from build123d import *

# Parameters (mm, degrees)
F1_DEPTH = 1.27
F2_DEPTH = 8.89
F3_R     = 5.715
F3_R_2   = 2.9972
F4_DEPTH = 1.27
F5_R     = 6.35
F5_R_2   = 2.9972
F6_DEPTH = 1.27


with BuildPart() as f1:
    # F0 (on Front) → F1 (new body)
    with BuildSketch(Plane.XZ):
        with BuildLine():
            ThreePointArc((7.62, 0), (5.388154, 5.388154), (0, 7.62))
            Line((0, 7.62), (0, 6.35))
            Line((0, 6.35), (3.683, 6.35))
            Line((3.683, 6.35), (7.315638, 0))
            Line((7.315638, 0), (7.62, 0))
        make_face()
        with BuildLine():
            Line((0, 6.35), (0, 7.62))
            ThreePointArc((0, 7.62), (-5.388154, 5.388154), (-7.62, 0))
            Line((-7.62, 0), (-7.315638, 0))
            Line((-7.315638, 0), (-3.683, 6.35))
            Line((-3.683, 6.35), (0, 6.35))
        make_face()
        with BuildLine():
            ThreePointArc((0, -7.62), (5.388154, -5.388154), (7.62, 0))
            Line((7.62, 0), (7.315638, 0))
            Line((7.315638, 0), (3.683, -6.35))
            Line((3.683, -6.35), (0, -6.35))
            Line((0, -6.35), (0, -7.62))
        make_face()
        with BuildLine():
            Line((-7.315638, 0), (-7.62, 0))
            ThreePointArc((-7.62, 0), (-5.388154, -5.388154), (0, -7.62))
            Line((0, -7.62), (0, -6.35))
            Line((0, -6.35), (-3.683, -6.35))
            Line((-3.683, -6.35), (-7.315638, 0))
        make_face()
    extrude(amount=F1_DEPTH)

    # F0 (on Front) → F2 (join)
    with BuildSketch(Plane.XZ):
        with BuildLine():
            Line((3.683, 6.35), (0, 6.35))
            Line((0, 6.35), (0, 2.9972))
            ThreePointArc((0, 2.9972), (2.11934, 2.11934), (2.9972, 0))
            Line((2.9972, 0), (7.315638, 0))
            Line((7.315638, 0), (3.683, 6.35))
        make_face()
        with BuildLine():
            Line((0, 2.9972), (0, 6.35))
            Line((0, 6.35), (-3.683, 6.35))
            Line((-3.683, 6.35), (-7.315638, 0))
            Line((-7.315638, 0), (-2.9972, 0))
            ThreePointArc((-2.9972, 0), (-2.11934, 2.11934), (0, 2.9972))
        make_face()
        with BuildLine():
            Line((-2.9972, 0), (-7.315638, 0))
            Line((-7.315638, 0), (-3.683, -6.35))
            Line((-3.683, -6.35), (0, -6.35))
            Line((0, -6.35), (0, -2.9972))
            ThreePointArc((0, -2.9972), (-2.11934, -2.11934), (-2.9972, 0))
        make_face()
        with BuildLine():
            Line((3.683, -6.35), (7.315638, 0))
            Line((7.315638, 0), (2.9972, 0))
            ThreePointArc((2.9972, 0), (2.11934, -2.11934), (0, -2.9972))
            Line((0, -2.9972), (0, -6.35))
            Line((0, -6.35), (3.683, -6.35))
        make_face()
    extrude(amount=F2_DEPTH)

    # F3 (on face) → F4 (join)
    with BuildSketch(Plane.XZ.offset(8.89)):
        Circle(F3_R)
        Circle(F3_R_2, mode=Mode.SUBTRACT)
    extrude(amount=F4_DEPTH)

    # F5 (on face) → F6 (join)
    with BuildSketch(Plane.XZ.offset(10.16)):
        Circle(F5_R)
        Circle(F5_R_2, mode=Mode.SUBTRACT)
    extrude(amount=F6_DEPTH)


solid = f1.part
Geometry check sheet. Reference: the model listing, model coordinates, mm. A direction names the side the tool comes from. Give positions to 0.01 mm unless a question says otherwise; leave off trailing zeros. Write each loop counter-clockwise with the first axis right and the second up, starting at its lowest first coordinate (ties: lowest second). Pieces come first, ordered by that corner, then holes. Notation, with made-up numbers: M 61.25,-31 L 68.25,-31 A21 ccw 68.25,-22 Z; hole C 23.5,35.5 d10. An arc over 180 degrees is marked long. Answer as CSV lines item,"result". Start each with the question number.
Q1. Go/stop test with flat-tipped pins: pin 1 (2 mm diameter, centred on x = 6, y = -1.5, fed in from -Z); pin 2 (3.5 mm diameter, centred on x = 0, y = -4, fed in from +Z); pin 3 (4 mm diameter, centred on y = -4.5, z = 5.5, fed in from -X). Record where each tip stops, or that it passes through.
Q2. Section check D-D, the plane x = 4.5. Record the cut outline in (y, z).
Q3. Section check B-B, the plane z = -1. Record the cut outline in (x, y), then the cut area to 3 significant figures.
Q4. Section check C-C, the plane x = 2.5. Record the cut outline in (y, z), then the cut area to 3 significant figures.
Q5. Material ranges on L1, parallel to Y at x = -5.75, z = -1.5; L2, parallel to Z at x = 0, y = -9.5 (3 decimals); L3, parallel to Z at x = 0, y = -10.85, recorded low to high.
Q6. Release check for a two-part mould opening along Y. For faces 4 (the face through (3, -11.43, -1)), 5 (the face through (4.84, -8.89, 3.32)), 6 (the face through (5.45, -9.52, 1.72)), 7 (the face through (0, -5, -6.35)) record: pulls with the +Y half, pulls with the -Y half, needs draft (parallel to the pull), parting line crosses it, or undercut.
Q7. Tool access check on faces 1 (the face through (-5.474, -5.027, 3.219)), 2 (the face through (-1.38, -10.79, -6.2)), 3 (the face through (5.525, -5.027, 3.131)). Record the directions out of +Z, -Z, +X, -X, +Y, -Y that give a thin tool (end or side, any length) a straight path to the whole face; none if there is none.
Q8. Section check A-A, the plane y = -1. Record the cut outline in (x, z).
Geometry says:
1,pin 1,"z = -5.73"
1,pin 2,"z = 6.35"
1,pin 3,"x = -5.31"
2,outline,"M -11.43,-4.48 L -10.16,-4.48 L -10.16,-3.52 L -8.89,-3.52 L -8.89,-4.92 L -1.27,-4.92 L -1.27,-6.15 L 0,-6.15 L 0,6.15 L -1.27,6.15 L -1.27,4.92 L -8.89,4.92 L -8.89,3.52 L -10.16,3.52 L -10.16,4.48 L -11.43,4.48 Z"
3,outline,"M -7.55,-1.27 L -6.74,-1.27 L -6.74,-8.89 L -5.63,-8.89 L -5.63,-10.16 L -6.27,-10.16 L -6.27,-11.43 L -2.83,-11.43 L -2.83,0 L -7.55,0 Z; M 2.83,-11.43 L 6.27,-11.43 L 6.27,-10.16 L 5.63,-10.16 L 5.63,-8.89 L 6.74,-8.89 L 6.74,-1.27 L 7.55,-1.27 L 7.55,0 L 2.83,0 Z"
3,area,"87.6 mm^2"
4,outline,"M -11.43,-5.84 L -10.16,-5.84 L -10.16,-5.14 L -8.89,-5.14 L -8.89,-6.35 L -1.27,-6.35 L -1.27,-7.2 L 0,-7.2 L 0,-1.65 L -11.43,-1.65 Z; M -11.43,1.65 L 0,1.65 L 0,7.2 L -1.27,7.2 L -1.27,6.35 L -8.89,6.35 L -8.89,5.14 L -10.16,5.14 L -10.16,5.84 L -11.43,5.84 Z"
4,area,"105 mm^2"
5,L1,"-11.43 to -10.16, -8.89 to 0"
5,L2,"-5.715 to -2.997, 2.997 to 5.715"
5,L3,"-6.35 to -3, 3 to 6.35"
6,face 4,"pulls with the -Y half"
6,face 5,"undercut"
6,face 6,"undercut"
6,face 7,"needs draft"
7,face 1,"+Z, -X, -Y"
7,face 2,"-Y"
7,face 3,"+Z, +X, -Y"
8,outline,"M -7.62,0 A7.62 ccw 0,-7.62 A7.62 ccw 7.62,0 A7.62 ccw 0,7.62 A7.62 ccw Z; hole M -3,0 A3 ccw 0,-3 A3 ccw 3,0 A3 ccw 0,3 A3 ccw Z"
